```python
from build123d import *

# Parameters (mm, degrees)
F0_W     = 25.4
F0_H     = 15.875
F1_DEPTH = 38.1
F2_R     = 4.7625
F3_DEPTH = 254000
F4_W     = 25.4
F4_H     = 12.7
F5_DEPTH = 35.56


with BuildPart() as f1:
    # F0 (on Top) → F1 (new body)
    with BuildSketch(Plane.XY):
        with Locations((-45.274386, -11.600519)):
            Rectangle(F0_W, F0_H)
    extrude(amount=F1_DEPTH)

    # F2 (on face) → F3 (cut)
    with BuildSketch(Plane.XZ.offset(19.538019)):
        with Locations((-45.274386, 22.86)):
            Circle(F2_R)
    extrude(amount=-F3_DEPTH, mode=Mode.SUBTRACT)

    # F4 (on face) → F5 (join)
    with BuildSketch(Plane(origin=(0, -3.663019, 0), x_dir=(-1, 0, 0), z_dir=(0, 1, 0))):
        with Locations((45.274386, 6.35)):
            Rectangle(F4_W, F4_H)
    extrude(amount=F5_DEPTH)


solid = f1.part
```
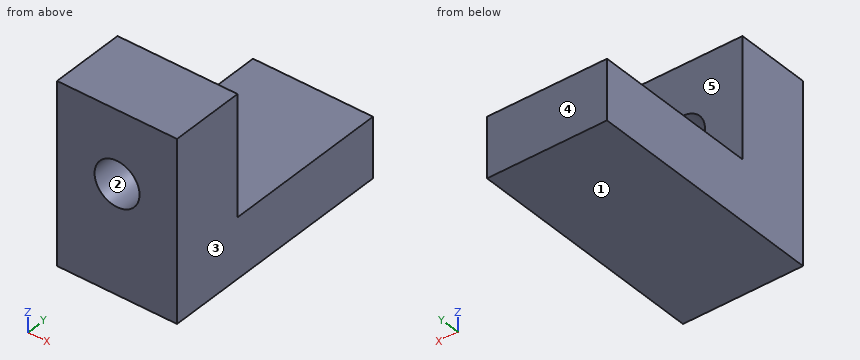
Geometry: final body of the model. Coordinates: model frame, mm. Face numbers are marked on the shaded views. A direction names the side the tool comes from. Round coordinates to 2 decimals unless told otherwise and drop trailing zeros. Order: outer loops, then holes, each group sorted by start corner. A loop starts at its lowest first (then second) coordinate and runs counter-clockwise, first axis right, second up. Notation, with made-up numbers: M 18,-8 L 33,-8 A11 ccw 33,9 Z; hole C 50.25,50.25 d2. An arc over 180 degrees is marked long. One line per item, written item: value.
(1) Line query: probe 1 along Y at (x, z) = (-34, 27); probe 2 along Z at (x, y) = (-55.5, 5); probe 3 along X at (y, z) = (-12, 22). Output: solid intervals per line, ascending. Write a range as [from, to].
Result sheet:
probe 1: [-19.54, -3.66]
probe 2: [0, 12.7]
probe 3: [-57.97, -49.96], [-40.59, -32.57]
(2) Reachability of the marked faces 4 and 5 from +Z, -Z, +X, -X, +Y, -Y: full face, straight path, thin tool, end or side. Return the list, or none.
Result sheet:
face 4: +Z, -Z, +X, -X, +Y
face 5: +Z, +X, -X, +Y
(3) Pull-direction query (Z, two-part tool) for the marked faces 1, 2 and 3; classes: pulls with the +Z half, pulls with the -Z half, needs draft (parallel to the pull), parting line crosses it, or undercut.
Result sheet:
face 1: pulls with the -Z half
face 2: undercut
face 3: needs draft
(4) Cut plane D-D (x = -54.5). Return the cut outline in (y, z).
Result sheet:
outline: M -19.54,0 L 31.9,0 L 31.9,12.7 L -3.66,12.7 L -3.66,38.1 L -19.54,38.1 Z
(5) Cut plane A-A (y = -11). Return the cut outline in (x, z) (1 decimal), and give its area (3 significant figures).
Result sheet:
outline: M -58,0 L -32.6,0 L -32.6,38.1 L -58,38.1 Z; hole C -45.3,22.9 d9.5
area: 896 mm2
(6) Cut plane B-B (z = 22.86). Return the cut outline in (x, y).
Result sheet:
outline: M -57.97,-19.54 L -50.04,-19.54 L -50.04,-3.66 L -57.97,-3.66 Z; M -40.51,-19.54 L -32.57,-19.54 L -32.57,-3.66 L -40.51,-3.66 Z
(7) Cut plane C-C (x = -48). Return the cut outline in (y, z).
Result sheet:
outline: M -19.54,0 L 31.9,0 L 31.9,12.7 L -3.66,12.7 L -3.66,18.95 L -19.54,18.95 Z; M -19.54,26.77 L -3.66,26.77 L -3.66,38.1 L -19.54,38.1 Z
(8) Pin query (flat end, axial travel): P1, Ø6, axis at y = 1, z = 34, coming from the +X side; P2, Ø12.5, axis at x = -43.5, y = 13.5, coming from the +Z side; P3, Ø2, axis at x = -38.5, z = 24.5, coming from the +Y side. Return the tip coordinate at first contact, or that it passes through.
Result sheet:
P1: through
P2: z = 12.7
P3: y = -3.66
